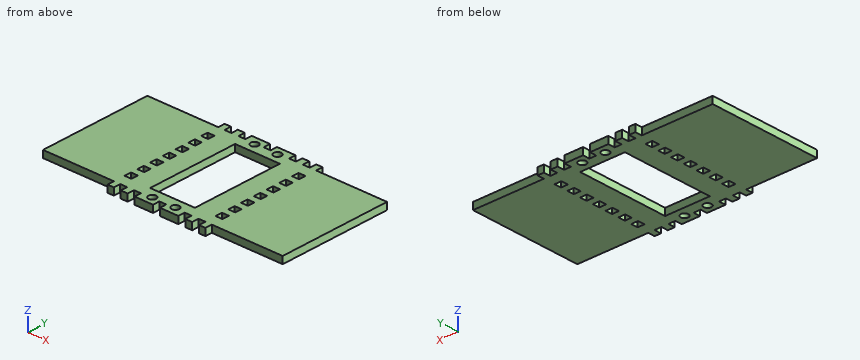
from build123d import *

# Parameters (mm, degrees)
F0_R     = 1.65
F0_W     = 19.4
F0_H     = 39.9
F1_DEPTH = 3
F3_DEPTH = 3


with BuildPart() as f1:
    # F0 (on Top) → F1 (new body)
    with BuildSketch(Plane.XY):
        Polygon((17.517377, -26.128115), (20.267377, -26.128115), (20.267377, -18.128115), (17.267377, -18.128115), (17.267377, -15.128115), (20.267377, -15.128115), (20.267377, -12.128115), (17.267377, -12.128115), (17.267377, -9.128115), (20.267377, -9.128115), (20.267377, -6.128115), (17.267377, -6.128115), (17.267377, -3.128115), (20.267377, -3.128115), (20.267377, -0.128115), (17.267377, -0.128115), (17.267377, 2.871885), (20.267377, 2.871885), (20.267377, 5.871885), (17.267377, 5.871885), (17.267377, 8.871885), (20.267377, 8.871885), (20.267377, 11.871885), (17.267377, 11.871885), (17.267377, 14.871885), (20.267377, 14.871885), (20.267377, 17.871885), (17.267377, 17.871885), (17.267377, 20.871885), (20.267377, 20.871885), (20.267377, 28.871885), (17.517377, 28.871885), (17.517377, 25.871885), (14.517377, 25.871885), (14.517377, 28.871885), (11.517377, 28.871885), (11.517377, 25.871885), (8.517377, 25.871885), (8.517377, 28.871885), (0.517377, 28.871885), (0.517377, 25.871885), (-2.482623, 25.871885), (-2.482623, 28.871885), (-10.482623, 28.871885), (-10.482623, 25.871885), (-13.482623, 25.871885), (-13.482623, 28.871885), (-16.482623, 28.871885), (-16.482623, 25.871885), (-19.482623, 25.871885), (-19.482623, 28.871885), (-22.232623, 28.871885), (-22.232623, 20.871885), (-19.232623, 20.871885), (-19.232623, 17.871885), (-22.232623, 17.871885), (-22.232623, 14.871885), (-19.232623, 14.871885), (-19.232623, 11.871885), (-22.232623, 11.871885), (-22.232623, 8.871885), (-19.232623, 8.871885), (-19.232623, 5.871885), (-22.232623, 5.871885), (-22.232623, 2.871885), (-19.232623, 2.871885), (-19.232623, -0.128115), (-22.232623, -0.128115), (-22.232623, -3.128115), (-19.232623, -3.128115), (-19.232623, -6.128115), (-22.232623, -6.128115), (-22.232623, -9.128115), (-19.232623, -9.128115), (-19.232623, -12.128115), (-22.232623, -12.128115), (-22.232623, -15.128115), (-19.232623, -15.128115), (-19.232623, -18.128115), (-22.232623, -18.128115), (-22.232623, -26.128115), (-19.482623, -26.128115), (-19.482623, -23.128115), (-16.482623, -23.128115), (-16.482623, -26.128115), (-13.482623, -26.128115), (-13.482623, -23.128115), (-10.482623, -23.128115), (-10.482623, -26.128115), (-2.482623, -26.128115), (-2.482623, -23.128115), (0.517377, -23.128115), (0.517377, -26.128115), (8.517377, -26.128115), (8.517377, -23.128115), (11.517377, -23.128115), (11.517377, -26.128115), (14.517377, -26.128115), (14.517377, -23.128115), (17.517377, -23.128115), align=None)
        with Locations((-5.982623, -22.628115)):
            Circle(F0_R, mode=Mode.SUBTRACT)
        with Locations((4.017377, -22.628115)):
            Circle(F0_R, mode=Mode.SUBTRACT)
        with Locations((-0.982623, 1.371885)):
            Rectangle(F0_W, F0_H, mode=Mode.SUBTRACT)
        with Locations((-5.982623, 25.371885)):
            Circle(F0_R, mode=Mode.SUBTRACT)
        with Locations((4.017377, 25.371885)):
            Circle(F0_R, mode=Mode.SUBTRACT)
    extrude(amount=F1_DEPTH)

    # F2 (on face) → F3 (join)
    with BuildSketch(Plane.XY.offset(3)):
        Polygon((-52.982623, -23.128115), (-22.232623, -23.128115), (-22.232623, -18.128115), (-22.232623, -15.128115), (-22.232623, -12.128115), (-22.232623, -9.128115), (-22.232623, -6.128115), (-22.232623, -3.128115), (-22.232623, -0.128115), (-22.232623, 2.871885), (-22.232623, 5.871885), (-22.232623, 8.871885), (-22.232623, 11.871885), (-22.232623, 14.871885), (-22.232623, 17.871885), (-22.232623, 20.871885), (-22.232623, 25.871885), (-52.982623, 25.871885), align=None)
        Polygon((20.267377, -18.128115), (20.267377, -23.128115), (51.017377, -23.128115), (51.017377, 25.871885), (20.267377, 25.871885), (20.267377, 20.871885), (20.267377, 17.871885), (20.267377, 14.871885), (20.267377, 11.871885), (20.267377, 8.871885), (20.267377, 5.871885), (20.267377, 2.871885), (20.267377, -0.128115), (20.267377, -3.128115), (20.267377, -6.128115), (20.267377, -9.128115), (20.267377, -12.128115), (20.267377, -15.128115), align=None)
    extrude(amount=-F3_DEPTH)


solid = f1.part
Geometry check sheet. Reference: the model listing, model coordinates, mm. Round coordinates to 2 decimals unless told otherwise and drop trailing zeros. Write each loop counter-clockwise with the first axis right and the second up, starting at its lowest first coordinate (ties: lowest second). Pieces come first, ordered by that corner, then holes. Notation, with made-up numbers: (18, -34) -> (74, -34) arc R19 ccw to (74, -11) -> close; hole circle Ø8 at (55.5, 25.25). An arc over 180 degrees is marked (long way). One line per item, written item: value. Start each with the question number.
(1) Scan lines: line 1 (X direction, y = 0, z = 2.4); line 2 (X direction, y = 11, z = 2.95); line 3 (Y direction, x = -10, z = 1.5). Record each from-to range of solid material in increasing order. Write a range as [from, to].
(2) Cross-section at C-C, the plane x = -41.5. Record the cut outline in (y, z).
(3) Cross-section at A-A, the plane y = -5. Record the cut outline in (x, z), and give its area (3 significant figures).
(4) Go/stop test with flat-tipped pins: pin 1 Ø0.9 at (y, z) = (-24.5, 2) entering from -X; pin 2 Ø1.5 at (x, z) = (-1, 1) entering from -Y; pin 3 Ø2.5 at (x, y) = (4.02, 25.37) entering from +Z. Record where each tip stops, or that it passes through.
(5) Cross-section at B-B, the plane x = -9. Record the cut outline in (y, z), and give its area (3 significant figures).
(6) Cross-section at D-D, the plane z = 0.6. Give the number of separate pieces and of enclosed holes in the cut face, and give its area (3 significant figures).
Answer:
1. line 1: [-52.98, -22.23], [-19.23, -10.68], [8.72, 17.27], [20.27, 51.02]
1. line 2: [-52.98, -10.68], [8.72, 51.02]
1. line 3: [-26.13, -18.58], [21.32, 28.87]
2. outline: (-23.13, 0) -> (25.87, 0) -> (25.87, 3) -> (-23.13, 3) -> close
3. outline: (-52.98, 0) -> (-22.23, 0) -> (-22.23, 3) -> (-52.98, 3) -> close; (-19.23, 0) -> (-10.68, 0) -> (-10.68, 3) -> (-19.23, 3) -> close; (8.72, 0) -> (17.27, 0) -> (17.27, 3) -> (8.72, 3) -> close; (20.27, 0) -> (51.02, 0) -> (51.02, 3) -> (20.27, 3) -> close
3. area: 236 mm²
4. pin 1: x = -22.23
4. pin 2: y = -23.13
4. pin 3: through
5. outline: (-26.13, 0) -> (-18.58, 0) -> (-18.58, 3) -> (-26.13, 3) -> close; (21.32, 0) -> (28.87, 0) -> (28.87, 3) -> (21.32, 3) -> close
5. area: 45.3 mm²
6. separate pieces: 1
6. enclosed holes: 19
6. area: 4,330 mm²
